```python
from build123d import *

# Parameters (mm, degrees)
F1_DEPTH = 200
F2_SIZE  = 100


with BuildPart() as f1:
    # F0 (on Right) → F1 (new body, symmetric)
    with BuildSketch(Plane.YZ):
        Polygon((-130, 0), (0, 0), (0, 350), (-3, 350), (-3, 3), (-130, 3), align=None)
    extrude(amount=F1_DEPTH, both=True)

    # F2
    f2_edges = [f1.edges().sort_by_distance(p)[0] for p in [
        (200, -1.5, 350),
        (-200, -1.5, 350),
    ]]
    chamfer(f2_edges, length=F2_SIZE)


solid = f1.part
```
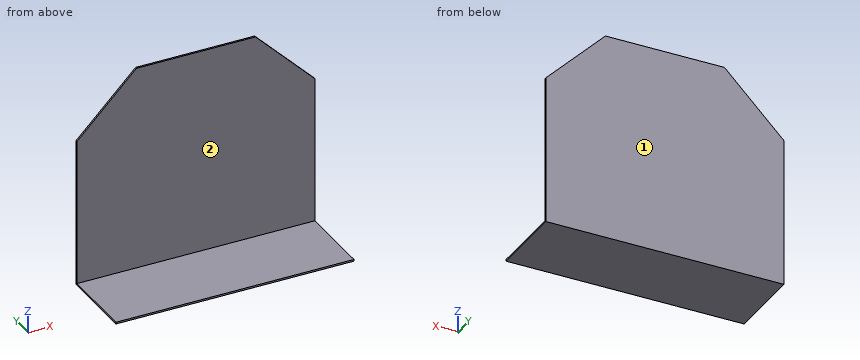
Read the model definition and answer for the solid it produces. Units are mm, in the model's axes. Face numbers are marked on the shaded views. A direction names the side the tool comes from. Coordinates: 2 decimals unless noted, no trailing zeros. Loops run counter-clockwise (first coordinate to the right, second up) from the corner with the lowest first, then second, coordinate; pieces in that order, holes last.
(1) Consider line 1 along Z through (x, y) = (18, -30.5); line 2 along Y through (x, z) = (-89, 226). Determine where each line is inside the solid, lowest interval first.
Solution:
line 1: z = 0 to 3
line 2: y = -3 to 0
(2) A tool of negligible diameter and unlimited length cuts with its end or side. For the marked faces 1 and 2, from which of +Z, -Z, +X, -X, +Y, -Y can it reach the whole face along a straight path? Write none if from no direction.
Solution:
face 1: +Z, -Z, +X, -X, +Y
face 2: +Z, +X, -X, -Y
(3) A flat-ended cylindrical pin translates along its axis: pin 1 Ø12 at (x, z) = (123, 252) entering from -Y. Find the tip coordinate at first contact, or state that the pin passes through.
Solution:
pin 1: stops at y = -3
(4) The part is cut by section A-A (x = 38). Determine the outline of the cut face in (y, z).
Solution:
outline: (-130, 0) - (0, 0) - (0, 350) - (-3, 350) - (-3, 3) - (-130, 3) - close
(5) The part is cut by section B-B (z = 270). Determine the outline of the cut face in (x, y).
Solution:
outline: (-180, -3) - (180, -3) - (180, 0) - (-180, 0) - close
(6) The part is cut by section C-C (y = -102). Determine the outline of the cut face in (x, z).
Solution:
outline: (-200, 0) - (200, 0) - (200, 3) - (-200, 3) - close
(7) The part is cut by section D-D (x = 155.5). Determine the outline of the cut face in (y, z), and give its area (3 significant figures).
Solution:
outline: (-130, 0) - (0, 0) - (0, 294.5) - (-3, 294.5) - (-3, 3) - (-130, 3) - close
area: 1,260 mm2
